Could you check a few things on this model? Use its own coordinates, in mm. Face numbers are marked on the shaded views. Coordinates: 2 decimals unless noted, no trailing zeros. Loops run counter-clockwise (first coordinate to the right, second up) from the corner with the lowest first, then second, coordinate; pieces in that order, holes last. Notation, with made-up numbers: (50, -32) - (94, -32) arc R16 cw to (94, -16) - close; hole circle Ø11 at (37, -10). An arc over 180 degrees is marked (long way). One line per question, with ' | ' between items. Start each with the question number.
1. I want a section at D-D, the plane z = -3.5. Write out the boundary of the cut face in (x, y) (1 decimal).
2. We'd pull the mould along Y, two halves only. Please class the marked faces 1, 2 and 3: pulls with the +Y half, pulls with the -Y half, needs draft (parallel to the pull), parting line crosses it, or undercut.
3. Please list where these lines run through material, in increasing order: L1, parallel to Y at x = 24.5, z = 10 (3 decimals); L2, parallel to Z at x = -24, y = 19.75; L3, parallel to X at y = 6, z = 18. Write a range as [from, to].
4. I want a section at A-A, the plane z = 9.25. Write out the boundary of the cut face in (x, y) (1 decimal).
5. I'm going to push flat-ended pins straight in: P1, Ø11, axis at x = 32.5, z = 8, coming from the -Y side; P2, Ø8, axis at y = 8.5, z = 8.5, coming from the +X side; P3, Ø5.5, axis at x = -17, y = 13.5, coming from the -Z side. Where does each tip first touch, or does it pass through?
6. I want a section at C-C, the plane y = 13.25. Write out the boundary of the cut face in (x, z), then the cut area to 3 significant figures.
7. I want a section at B-B, the plane x = -58. Write out the boundary of the cut face in (y, z) (3 decimals).
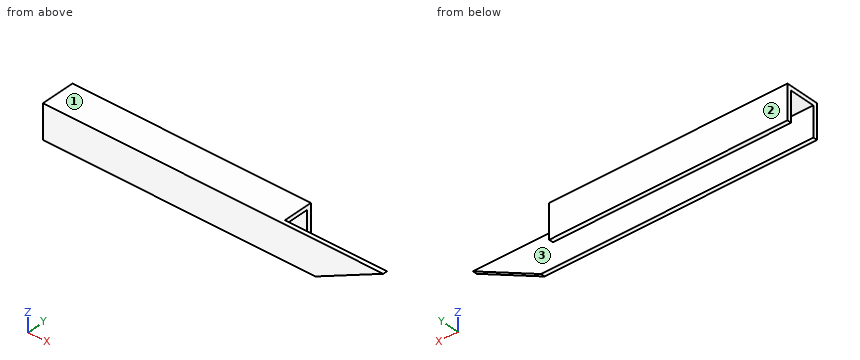
from build123d import *

# Parameters (mm, degrees)
BOSS_EXTRUDE1_DEPTH = 25.4
SKETCH2_W           = 19.05
SKETCH2_H           = 19.05
CUT_EXTRUDE1_DEPTH  = 257.020099216
CUT_EXTRUDE2_DEPTH  = 22.225
SKETCH5_W           = 177.8
SKETCH5_H           = 19.05
CUT_EXTRUDE4_DEPTH  = 22.225


with BuildPart() as part:
    # Sketch1 → Boss-Extrude1 (new body)
    with BuildSketch(Plane(origin=(0, 0, 0), x_dir=(1, 0, 0), z_dir=(0, 1, 0))):
        Polygon((-78.640492639, -19.624759931), (175.359507361, -19.624759931), (124.559507361, 5.775240069), (-78.640492639, 5.775240069), align=None)
    extrude(amount=BOSS_EXTRUDE1_DEPTH)

    # Sketch2 → Cut-Extrude1 (cut, through all)
    with BuildSketch(Plane.ZY.offset(78.640492639)):
        with Locations((6.924759931, 12.7)):
            Rectangle(SKETCH2_W, SKETCH2_H)
    extrude(amount=-CUT_EXTRUDE1_DEPTH, mode=Mode.SUBTRACT)

    # Sketch3 → Cut-Extrude2 (cut)
    with BuildSketch(Plane(origin=(0, 25.4, 0), x_dir=(1, 0, 0), z_dir=(0, 1, 0))):
        Polygon((99.159507361, 5.775240069), (99.159507361, -19.624759931), (175.359507361, -19.624759931), (124.559507361, 5.775240069), align=None)
    extrude(amount=-CUT_EXTRUDE2_DEPTH, mode=Mode.SUBTRACT)

    # Sketch5 → Cut-Extrude4 (cut)
    with BuildSketch(Plane(origin=(0, 0, -5.775240069), x_dir=(-1, 0, 0), z_dir=(0, 0, -1))):
        with Locations((-10.259507361, 12.7)):
            Rectangle(SKETCH5_W, SKETCH5_H)
    extrude(amount=-CUT_EXTRUDE4_DEPTH, mode=Mode.SUBTRACT)


solid = part.part
Results are:
1) outline: (-78.6, 0) - (129.1, 0) - (129.1, 3.2) - (-78.6, 3.2) - close; (-78.6, 22.2) - (99.2, 22.2) - (99.2, 25.4) - (-78.6, 25.4) - close
2) face 1: needs draft | face 2: pulls with the +Y half | face 3: undercut
3) L1: y = [0, 3.175], [22.225, 25.4] | L2: z = [16.45, 19.62] | L3: x = [-78.64, 99.16]
4) outline: (-78.6, 0) - (154.6, 0) - (154.6, 3.2) - (-78.6, 3.2) - close; (-78.6, 22.2) - (99.2, 22.2) - (99.2, 25.4) - (-78.6, 25.4) - close
5) P1: stops at y = 0 | P2: passes through | P3: stops at z = 16.45
6) outline: (-78.64, 16.45) - (99.16, 16.45) - (99.16, 19.62) - (-78.64, 19.62) - close | area: 565 mm2
7) outline: (0, -5.775) - (3.175, -5.775) - (3.175, 16.45) - (22.225, 16.45) - (22.225, -5.775) - (25.4, -5.775) - (25.4, 19.625) - (0, 19.625) - close
